Geometry check sheet. Reference: drawing and pictorial views, mm from the part's lowest x, y, z. A direction names the side the tool comes from. Give positions to 0.01 mm unless a question says otherwise; leave off trailing zeros. Loops run counter-clockwise (first coordinate to the right, second up) from the corner with the lowest first, then second, coordinate; pieces in that order, holes last. Notation, with made-up numbers: (27.5, 62) -> (55.5, 62) arc R11 ccw to (55.5, 81) -> close; hole circle Ø11 at (72.5, -11). An arc over 180 degrees is marked (long way). Write each question's results on one line, items separated by ' | '. Start each with the question number.
1. Gauge pin test, flat ends, axial feed: pin 1 Ø3 at (x, y) = (27.5, 17.5) entering from +Z; pin 2 Ø1 at (x, y) = (34, 28) entering from -Z; pin 3 Ø1.5 at (x, z) = (26, 37.5) entering from +Y. Record the tip position at first contact, or that the pin passes through.
2. Cross-section at A-A on y = 20. Record the boundary of the cut face in (x, z).
3. Cross-section at C-C on z = 131. Record the boundary of the cut face in (x, y), and give its area (3 significant figures).
4. Tool access check on the marked faces 1, 2 and 3. Record the directions out of +Z, -Z, +X, -X, +Y, -Y that give a thin tool (end or side, any length) a straight path to the whole face; none if there is none.
5. Material ranges on L1, parallel to Z at x = 29, y = 16; L2, parallel to Y at x = 21, z = 99; L3, parallel to X at y = 9, z = 30, recorded low to high. Write a range as from..to.
6. Cross-section at D-D on z = 80. Record the boundary of the cut face in (x, y).
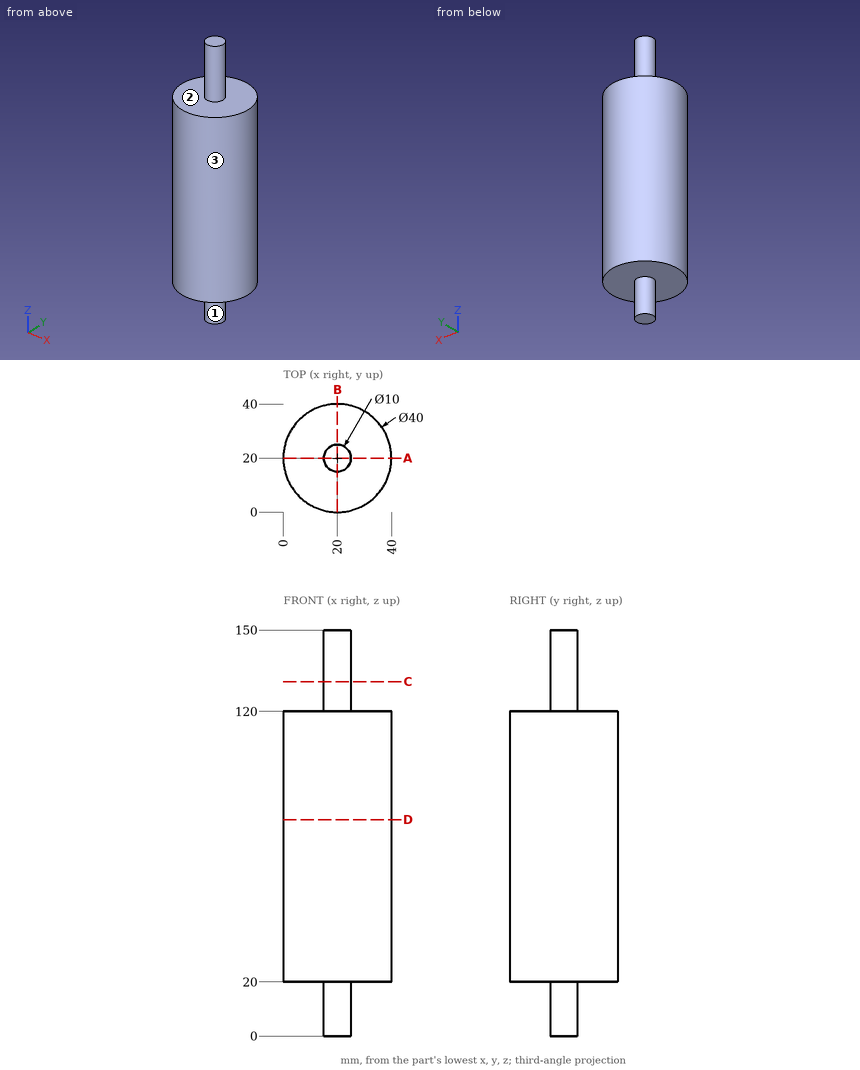
Geometry says:
1) pin 1: z = 120 | pin 2: z = 20 | pin 3: y = 39.3
2) outline: (0, 20) -> (15, 20) -> (15, 0) -> (25, 0) -> (25, 20) -> (40, 20) -> (40, 120) -> (25, 120) -> (25, 150) -> (15, 150) -> (15, 120) -> (0, 120) -> close
3) outline: circle Ø10 at (20, 20) | area: 78.5 mm^2
4) face 1: -Z | face 2: +Z | face 3: +Z, -Z
5) L1: 20..120 | L2: 0.03..39.97 | L3: 3.3..36.7
6) outline: circle Ø40 at (20, 20)
